Read the model definition and answer for the solid it produces. Units are mm, in the model's axes. A direction names the side the tool comes from. Coordinates: 2 decimals unless noted, no trailing zeros. Order: outer loops, then holes, each group sorted by start corner. A loop starts at its lowest first (then second) coordinate and runs counter-clockwise, first axis right, second up. Notation, with made-up numbers: (80.25, 78) -> (116.25, 78) arc R30 ccw to (116.25, 111) -> close; hole circle Ø9 at (32.25, 7). An arc over 180 degrees is marked (long way). Answer in a Markdown table with one row per item.
from build123d import *

# Parameters (mm, degrees)
EXTRUDE_2_DEPTH     = 8
SKETCH_5_W          = 24
SKETCH_5_H          = 35
EXTRUDE_3_DEPTH     = 27
CUT_EXTRUDE_1_DEPTH = 27


with BuildPart() as part:
    # 草图4 → 凸台-拉伸2 (new body)
    with BuildSketch(Plane(origin=(0, 0, 0), x_dir=(1, 0, 0), z_dir=(0, 1, 0))):
        Polygon((-12, 17.5), (-37, 8.5), (-37, 5.5), (-26, 5.5), (-26, -5.5), (-37, -5.5), (-37, -8.5), (-12, -17.5), (12, -17.5), (12, 17.5), align=None)
    extrude(amount=EXTRUDE_2_DEPTH)

    # 草图5 → 凸台-拉伸3 (add)
    with BuildSketch(Plane(origin=(0, 8, 0), x_dir=(1, 0, 0), z_dir=(0, 1, 0))):
        Rectangle(SKETCH_5_W, SKETCH_5_H)
    extrude(amount=EXTRUDE_3_DEPTH)

    # 草图6 → 切除-拉伸1 (cut)
    with BuildSketch(Plane.ZY.offset(12)):
        Polygon((-11.5, 35), (-5.5, 24), (-5.5, 18), (5.5, 18), (5.5, 24), (11.5, 35), align=None)
    extrude(amount=-CUT_EXTRUDE_1_DEPTH, mode=Mode.SUBTRACT)


solid = part.part
Q1. The part is cut by section D-D (x = 8.5). Write down the section's boundary in (y, z), then the cut area to 3 significant figures.
Outcome:
| item | result |
|---|---|
| outline | (0, -17.5) -> (35, -17.5) -> (35, -11.5) -> (24, -5.5) -> (18, -5.5) -> (18, 5.5) -> (24, 5.5) -> (35, 11.5) -> (35, 17.5) -> (0, 17.5) -> close |
| area | 972 mm² |
Q2. The part is cut by section B-B (y = 19.5). Write down the section's boundary in (x, z).
Outcome:
| item | result |
|---|---|
| outline | (-12, -17.5) -> (12, -17.5) -> (12, -5.5) -> (-12, -5.5) -> close; (-12, 5.5) -> (12, 5.5) -> (12, 17.5) -> (-12, 17.5) -> close |
Q3. For faces 4 (the face through (-22, 8, 0)), 5 (the face through (0, 18, 0)), 6 (the face through (-26, 4, 0)), 7 (the face through (-37, 4, -7)), 8 (the face through (0, 17, -17.5)), determine the directions among +Z, -Z, +X, -X, +Y, -Y from which every point of the face is accessible in a straight line to the end or side of a thin tool.
Outcome:
| item | result |
|---|---|
| face 4 | +Z, -Z, -X, +Y |
| face 5 | +X, -X, +Y |
| face 6 | -X, +Y, -Y |
| face 7 | +Z, -Z, -X, +Y, -Y |
| face 8 | -Z, +X, -X, +Y, -Y |
Q4. Consider line 1 (Z direction, x = 0, y = 23); line 2 (Y direction, x = -9.5, z = -3.5); line 3 (X direction, y = 15.5, z = -4). Determine where each line is inside the solid, lowest interval first.
Outcome:
| item | result |
|---|---|
| line 1 | -17.5 to -5.5, 5.5 to 17.5 |
| line 2 | 0 to 18 |
| line 3 | -12 to 12 |
Q5. For a pull along Z with two mould halves and no side action, classify faces 1 (the face through (0, 35, -15)), 2 (the face through (0, 17, 17.5)), 3 (the face through (-0.168, 29.423, 8.458)) as pulls with the +Z half, pulls with the -Z half, needs draft (parallel to the pull), parting line crosses it, or undercut.
Outcome:
| item | result |
|---|---|
| face 1 | needs draft |
| face 2 | pulls with the +Z half |
| face 3 | undercut |
Q6. Given pin 1 (7.5 mm diameter, centred on x = -23.5, z = -3.5, fed in from +Y); pin 2 (3 mm diameter, centred on y = 21, z = -13.5, fed in from -X); pin 3 (6.5 mm diameter, centred on y = 5.5, z = 1.5, fed in from -X), each flat-ended and moving along its own axis, determine where each tip first touches the part or whether it passes through.
Outcome:
| item | result |
|---|---|
| pin 1 | y = 8 |
| pin 2 | x = -12 |
| pin 3 | x = -26 |
Q7. The part is cut by section A-A (x = -28.5). Write down the section's boundary in (y, z).
Outcome:
| item | result |
|---|---|
| outline | (0, -11.56) -> (8, -11.56) -> (8, -5.5) -> (0, -5.5) -> close; (0, 5.5) -> (8, 5.5) -> (8, 11.56) -> (0, 11.56) -> close |
Q8. The part is cut by section C-C (z = 0). Write down the section's boundary in (x, y), then the cut area to 3 significant figures.
Outcome:
| item | result |
|---|---|
| outline | (-26, 0) -> (12, 0) -> (12, 18) -> (-12, 18) -> (-12, 8) -> (-26, 8) -> close |
| area | 544 mm² |
